Here's the drawing with two shaded views (mm, measured from the low corner). I have some questions. A direction names the side the tool comes from. Give positions to 0.01 mm unless a question says otherwise; leave off trailing zeros. Loops run counter-clockwise (first coordinate to the right, second up) from the corner with the lowest first, then second, coordinate; pieces in that order, holes last. Notation, with made-up numbers: (55, 8) -> (72, 8) arc R19 ccw to (72, 21) -> close; hole circle Ø9 at (61.25, 51.5). An arc over 180 degrees is marked (long way). Write each question's results on one line, items separated by ' | '. Start each with the question number.
Q1. Will this pin go through, and if not, where does the flat tip stop? P1, Ø1, axis at y = 13, z = 1, coming from the -X side.
Q2. If I drill on line 1 along Y through (x, z) = (3.5, 0.8); line 2 along Y through (x, z) = (7.5, 0.2); line 3 along X through (y, z) = (13, 0.9), over which ranges is the centre line in solid material (lowest first)?
Q3. Which directions (+Z, -Z, +X, -X, +Y, -Y) give clear straight access to the entire face, cutting with the end or side of a thin tool? Please do the marked faces 1 and 2.
Q4. If we section it at C-C, the plane y = 5.5: List the corners of the cut face in (x, z) for me.
Q5. If we section it at D-D, the plane x = 9: List the corners of the cut face in (y, z) for me.
Q6. If we section it at B-B, the plane x = 6.5: List the corners of the cut face in (y, z) for me.
Q7. We'd pull the mould along Y, two halves only. Please class the marked faces 3, 4 and 5: released by +Y, released by -Y, zero draft, split by the parting line, or undercut.
Q8. If we section it at A-A, the plane z = 0.95: List the corners of the cut face in (x, y) for me.
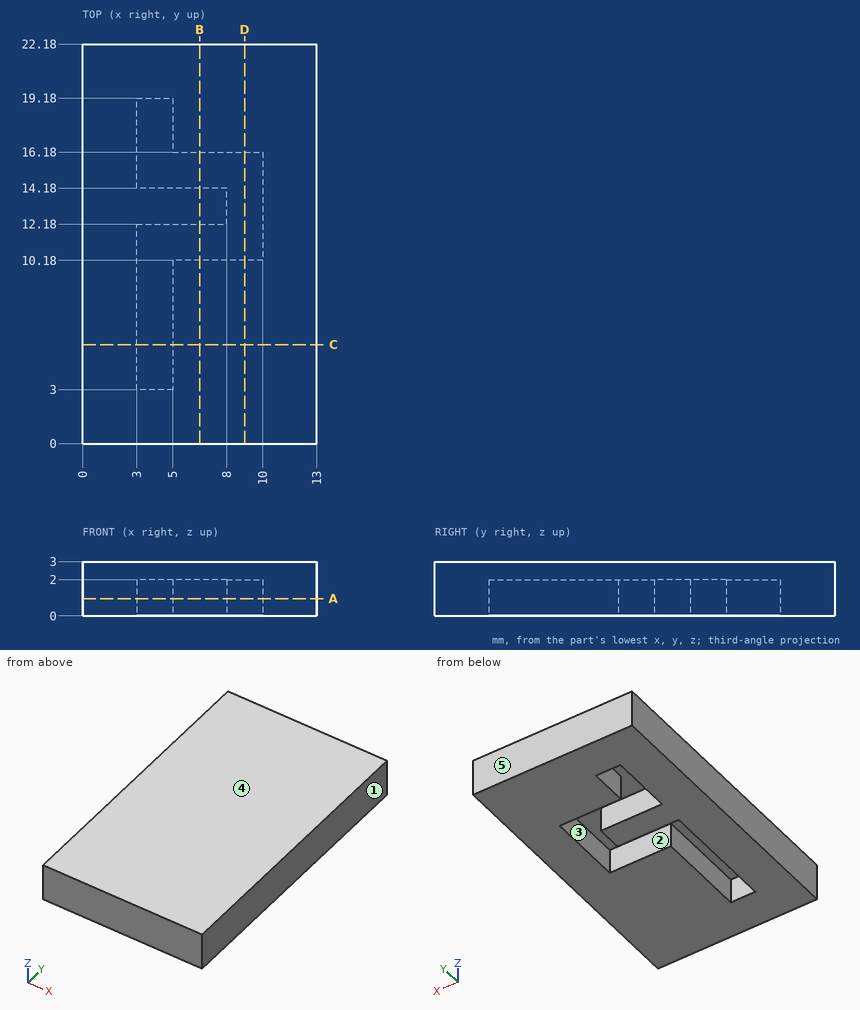
Final values:
1) P1: stops at x = 0
2) line 1: y = 0 to 3, 12.18 to 14.18, 19.18 to 22.18 | line 2: y = 0 to 10.18, 12.18 to 14.18, 16.18 to 22.18 | line 3: x = 0 to 8, 10 to 13
3) face 1: +Z, -Z, +X, +Y, -Y | face 2: -Z
4) outline: (0, 0) -> (3, 0) -> (3, 2) -> (5, 2) -> (5, 0) -> (13, 0) -> (13, 3) -> (0, 3) -> close
5) outline: (0, 0) -> (10.18, 0) -> (10.18, 2) -> (16.18, 2) -> (16.18, 0) -> (22.18, 0) -> (22.18, 3) -> (0, 3) -> close
6) outline: (0, 0) -> (10.18, 0) -> (10.18, 2) -> (12.18, 2) -> (12.18, 0) -> (14.18, 0) -> (14.18, 2) -> (16.18, 2) -> (16.18, 0) -> (22.18, 0) -> (22.18, 3) -> (0, 3) -> close
7) face 3: undercut | face 4: zero draft | face 5: released by +Y
8) outline: (0, 0) -> (13, 0) -> (13, 22.18) -> (0, 22.18) -> close; hole (3, 3) -> (5, 3) -> (5, 10.18) -> (10, 10.18) -> (10, 16.18) -> (5, 16.18) -> (5, 19.18) -> (3, 19.18) -> (3, 14.18) -> (8, 14.18) -> (8, 12.18) -> (3, 12.18) -> close
